from build123d import *

# Parameters (mm, degrees)
SKETCH1_R           = 37.5
BOSS_EXTRUDE1_DEPTH = 4
SKETCH2_R           = 1.75
CUT_EXTRUDE1_DEPTH  = 1
SKETCH3_R           = 35
CUT_EXTRUDE5_DEPTH  = 2.5
SKETCH4_R           = 17.5
CUT_EXTRUDE6_DEPTH  = 54.091901454


with BuildPart() as part:
    # Sketch1 → Boss-Extrude1 (new body)
    with BuildSketch(Plane(origin=(0, 0, 0), x_dir=(1, 0, 0), z_dir=(0, 1, 0))):
        with Locations(Location((0, 0, 0), (0, 0, 270))):
            Circle(SKETCH1_R)
    extrude(amount=BOSS_EXTRUDE1_DEPTH)

    # Sketch2 → Cut-Extrude1 (cut)
    with BuildSketch(Plane(origin=(0, 4, 0), x_dir=(1, 0, 0), z_dir=(0, 1, 0))):
        with Locations(Location((0, 30, 0), (0, 0, 270))):
            Circle(SKETCH2_R)
        with Locations(Location((30, 0, 0), (0, 0, 270))):
            Circle(SKETCH2_R)
        with Locations(Location((0, -30, 0), (0, 0, 270))):
            Circle(SKETCH2_R)
        with Locations(Location((-30, 0, 0), (0, 0, 270))):
            Circle(SKETCH2_R)
    extrude(amount=-CUT_EXTRUDE1_DEPTH, mode=Mode.SUBTRACT)

    # Sketch3 → Cut-Extrude5 (cut)
    with BuildSketch(Plane(origin=(0, 0, 0), x_dir=(-1, 0, 0), z_dir=(0, -1, 0))):
        with Locations(Location((0, 0, 0), (0, 0, 90))):
            Circle(SKETCH3_R)
    extrude(amount=-CUT_EXTRUDE5_DEPTH, mode=Mode.SUBTRACT)

    # Sketch4 → Cut-Extrude6 (cut, through all)
    with BuildSketch(Plane(origin=(0, 2.5, 0), x_dir=(-1, 0, 0), z_dir=(0, -1, 0))):
        with Locations(Location((0, 0, 0), (0, 0, 90))):
            Circle(SKETCH4_R)
    extrude(amount=-CUT_EXTRUDE6_DEPTH, mode=Mode.SUBTRACT)


solid = part.part
Input: part model. Units: mm. Frame: model coordinates. A direction names the side the tool comes from. Round coordinates to 2 decimals unless told otherwise and drop trailing zeros. Order: outer loops, then holes, each group sorted by start corner. A loop starts at its lowest first (then second) coordinate and runs counter-clockwise, first axis right, second up.
1. Cut plane B-B, the plane x = 15. Output: boundary loops of the cut face in (y, z), then the cut area to 3 significant figures.
The answers:
outline: (0, -34.37) - (4, -34.37) - (4, -9.01) - (2.5, -9.01) - (2.5, -31.62) - (0, -31.62) - close; (0, 31.62) - (2.5, 31.62) - (2.5, 9.01) - (4, 9.01) - (4, 34.37) - (0, 34.37) - close
area: 89.8 mm2
2. Material intervals for line 1 (Z direction, x = 1, y = 1.1); line 2 (Y direction, x = 17.5, z = -23); line 3 (Z direction, x = 7, y = 2.85), sorted ascending.
The answers:
line 1: z = -37.49 to -34.99, 34.99 to 37.49
line 2: y = 2.5 to 4
line 3: z = -36.84 to -16.04, 16.04 to 36.84
3. Cut plane D-D, the plane x = -22. Output: boundary loops of the cut face in (y, z), then the cut area to 3 significant figures.
The answers:
outline: (0, -30.37) - (4, -30.37) - (4, 30.37) - (0, 30.37) - (0, 27.22) - (2.5, 27.22) - (2.5, -27.22) - (0, -27.22) - close
area: 107 mm2
4. Cut plane C-C, the plane y = 1.2. Output: boundary loops of the cut face in (x, z), then the cut area to 3 significant figures.
The answers:
outline: circle Ø75 at (0, 0); hole circle Ø70 at (0, 0)
area: 569 mm2
5. Set-up query: faces 1 (the face through (-21, 1, 28)), 2 (the face through (30, 3, 0)), 3 (the face through (-10.648, 3.24, 13.887)). Return all of +Z, -Z, +X, -X, +Y, -Y with unobstructed straight access to the full face (end or side cutting, diameter ignored); none if empty.
The answers:
face 1: -Y
face 2: +Y
face 3: +Y, -Y
6. Pin query (flat end, axial travel): P1, Ø2, axis at x = -12, y = 2, coming from the -Z side; P2, Ø10, axis at x = -12, z = -22, coming from the -Y side; P3, Ø2, axis at y = 1.5, z = 18, coming from the +X side. Return the tip coordinate at first contact, or that it passes through.
The answers:
P1: stops at z = -35.85
P2: stops at y = 2.5
P3: stops at x = 33.43
7. Cut plane A-A, the plane z = 14. Output: boundary loops of the cut face in (x, y).
The answers:
outline: (-34.79, 0) - (-32.08, 0) - (-32.08, 2.5) - (-10.5, 2.5) - (-10.5, 4) - (-34.79, 4) - close; (10.5, 2.5) - (32.08, 2.5) - (32.08, 0) - (34.79, 0) - (34.79, 4) - (10.5, 4) - close
8. Mould query, pull axis X, two halves, no side actions, for faces 4 (the face through (-22.818, 1.972, -29.759)), 5 (the face through (0, 3, -30)), 6 (the face through (-16, 4, 8)), 7 (the face through (0.08, 3.51, -31.75)). Classes: released by +X, released by -X, zero draft, split by the parting line, or undercut.
The answers:
face 4: split by the parting line
face 5: undercut
face 6: zero draft
face 7: undercut
